```python
from build123d import *

# Parameters (mm, degrees)
F0_W     = 12.7
F0_H     = 6.35
F1_DEPTH = 17.78


with BuildPart() as f1:
    # F0 (on Top) → F1 (new body)
    with BuildSketch(Plane.XY):
        with Locations((6.35, 3.175)):
            Rectangle(F0_W, F0_H)
        Polygon((0, 0), (0, 6.35), (-6.35, 17.348523), (-11.849261, 14.173523), (-5.499261, 3.175), align=None)
        Polygon((-6.35, -10.998523), (0, 0), (-5.499261, 3.175), (-11.849261, -7.823523), align=None)
    extrude(amount=F1_DEPTH)


solid = f1.part
```
The listing builds one solid part. Answer for the finished solid, in the listing's coordinates (mm). A direction names the side the tool comes from. Coordinates: 2 decimals unless noted, no trailing zeros. Loops run counter-clockwise (first coordinate to the right, second up) from the corner with the lowest first, then second, coordinate; pieces in that order, holes last. Notation, with made-up numbers: M 16.25,3.5 L 65.25,3.5 A18 ccw 65.25,26.5 Z; hole C 76.25,86 d8. An arc over 180 degrees is marked long. Answer as CSV lines item,"result". Start each with the question number.
(1) The part is cut by section A-A (z = 10). Give the vertices of the cut face in (x, y) (3 decimals).
(2) For faces 1 (the flat face through (6, 6.35, 9)), 2 (the flat face through (12.7, 3, 9)), determine the directions among +Z, -Z, +X, -X, +Y, -Y from which every point of the face is accessible in a straight line to the end or side of a thin tool.
(3) Find the intervals of material crossed by L1, parallel to Y at x = -7.75, z = 17.25; L2, parallel to Y at x = 0.25, z = 8.5; L3, parallel to X at y = -2.5, z = 14.5, in increasing order. Write a range as [from, to].
(4) The part is cut by section B-B (x = 5). Give the vertices of the cut face in (y, z).
(5) The mould has two halves that part along Y. Classify faces 3 (the flat face through (-9.061, 15.783, 8.766)), 4 (the flat face through (6, 0, 9)), 5 (the flat face through (-8.72, 8.75, 8.77)), 6 (the flat face through (-8.63, -2.25, 8.77)): pulls with the +Y half, pulls with the -Y half, needs draft (parallel to the pull), parting line crosses it, or undercut.
(6) Given pin 1 (1 mm diameter, centred on y = 8.5, z = 4, fed in from +X); pin 2 (1 mm diameter, centred on y = -3, z = 13, fed in from +X); pin 3 (3 mm diameter, centred on x = -8.5, y = 3, fed in from -Z); pin 4 (4 mm diameter, centred on y = 8.5, z = 10.5, fed in from +X), each flat-ended and moving along its own axis, determine where each tip first touches the part or whether it passes through.
(7) The part is cut by section C-C (y = 4.75). Give the vertices of the cut face in (x, z), and give its area (3 significant figures).
Determined:
1,outline,"M -11.849,-7.824 L -6.35,-10.999 L 0,0 L 12.7,0 L 12.7,6.35 L 0,6.35 L -6.35,17.349 L -11.849,14.174 L -5.499,3.175 Z"
2,face 1,"+Z, -Z, +X, +Y"
2,face 2,"+Z, -Z, +X, +Y, -Y"
3,L1,"[-10.19, -0.72], [7.07, 16.54]"
3,L2,"[0, 6.35]"
3,L3,"[-8.78, -1.44]"
4,outline,"M 0,0 L 6.35,0 L 6.35,17.78 L 0,17.78 Z"
5,face 3,"pulls with the +Y half"
5,face 4,"pulls with the -Y half"
5,face 5,"undercut"
5,face 6,"undercut"
6,pin 1,"x = -0.95"
6,pin 2,"x = -1.44"
6,pin 3,"through"
6,pin 4,"x = -0.09"
7,outline,"M -6.41,0 L 12.7,0 L 12.7,17.78 L -6.41,17.78 Z"
7,area,"340 mm2"
